Autodesk Inventor part; units mm, degrees
ref_plane "YZ Plane" through (0, 0, 0) normal (1, 0, 0) x (0, 1, 0)
ref_plane "XZ Plane" through (0, 0, 0) normal (0, 1, 0) x (-1, 0, 0)
ref_plane "XY Plane" through (0, 0, 0) normal (0, 0, 1) x (1, 0, 0)
sketch "Sketch1" plane through (0, 0, 0) normal (0, 0, 1) x (1, 0, 0)
  line L0 (0, 0) -> (16, 0)
  line L1 (16, 0) -> (16, 16)
  line L2 (16, 16) -> (0, 16)
  line L3 (0, 16) -> (0, 0)
  dimension "d0" = 16
  dimension "d1" = 16
extrude "Extrusion1" add sketch "Sketch1" along normal blind 12
sketch "Sketch3" plane through (0, 0, 0) normal (0, -1, 0) x (1, 0, 0)
  line L0 (0, 0) -> (16, 0)
  line L1 (0, 0) -> (0, 12)
  circle A0 centre (6, 3) radius 0.75
  circle A1 centre (12.25, 6) radius 3.05
  dimension "d10" = 6.1
  dimension "d11" = 1.5
  dimension "d12" = 3
  dimension "d13" = 6
  dimension "d14" = 6
  dimension "d15" = 12.25
sketch "Sketch2" plane through (0, 0, 12) normal (0, 0, 1) x (1, 0, 0)
  line L0 (0, 16) -> (0, 0)
  circle A0 centre (6, 8) radius 3
  circle A1 centre (13.5, 8) radius 1.4
  point P0 (0, 8)
  dimension "d4" = 13.5
  dimension "d5" = 6
  dimension "d6" = 6
  dimension "d7" = 2.8
chamfer "Chamfer1" distance 0.5 angle 45 12 edges at (0, 0, 6) (8, 0, 12) (0, 8, 12) (8, 16, 12) (0, 16, 6) (0, 8, 0) (8, 16, 0) (8, 0, 0) (16, 8, 0) (16, 8, 12) (16, 0, 6) (16, 16, 6)
extrude "Extrusion4" cut sketch "Sketch3" against normal up to next
extrude "Extrusion5" cut sketch "Sketch2" against normal up to next
thread "Thread1"
thread "Thread2"
properties part number "E3D_Heaterblock"
CAD build for the part. Positions are in the model's coordinates, mm. A direction names the side the tool comes from. Round coordinates to 2 decimals unless told otherwise and drop trailing zeros. Loops run counter-clockwise (first coordinate to the right, second up) from the corner with the lowest first, then second, coordinate; pieces in that order, holes last. Notation, with made-up numbers: M -31.5,15.25 L 25.5,15.25 A23 cw 25.5,49.25 Z; hole C 70.25,15 d1. An arc over 180 degrees is marked long. Use a Markdown table: item, result. Add a question column.
(1) Cut at C-C (y = 11.75). Give the cut face in (x, z), and give its area (3 significant figures).
(2) Cut at D-D (x = 13.5). Give the cut face in (y, z).
(3) Cut at A-A (z = 6). Give the cut face in (x, y), and give its area (3 significant figures).
(4) Which spindle directions (+Z, -Z, +X, -X, +Y, -Y) get a long thin tool onto all of the face, cutting with end or side? Do faces 1 (the face through (16, 8, 6)), 2 (the face through (14.835, 8.421, 10.285)). Say none if no direction does.
(5) Drill centre lines: line 1 (Y direction, x = 6, z = 6.25); line 2 (Z direction, x = 6, y = 3.6); line 3 (Y direction, x = 6.75, z = 2). Where is each one in solid material? Low to high.
(6) Pull direction Y, two halves, no side cores. Call faces 3 (the face through (6, 0, 6)), 4 (the face through (6, 16, 6)), 5 (the face through (7.384, 5.338, 6.084)), 6 (the face through (10, 8, 0)): +Y half, -Y half, draft (parallel to the pull), parting line (faces both ways), or undercut.
(7) Cut at B-B (x = 6). Give the cut face in (y, z).
Geometry says:
| question | item | result |
|---|---|---|
| 1 | outline | M 0,0.5 L 0.5,0 L 15.5,0 L 16,0.5 L 16,11.5 L 15.5,12 L 0.5,12 L 0,11.5 Z; hole C 6,3 d1.5; hole C 12.25,6 d6.1 |
| 1 | area | 161 mm² |
| 2 | outline | M 0,0.5 L 0.5,0 L 15.5,0 L 16,0.5 L 16,3.22 L 0,3.22 Z; M 0,8.78 L 6.6,8.78 L 6.6,12 L 0.5,12 L 0,11.5 Z; M 9.4,8.78 L 16,8.78 L 16,11.5 L 15.5,12 L 9.4,12 Z |
| 3 | outline | M 0,0.5 L 0.5,0 L 9.2,0 L 9.2,16 L 0.5,16 L 0,15.5 Z; M 15.3,0 L 15.5,0 L 16,0.5 L 16,15.5 L 15.5,16 L 15.3,16 Z; hole C 6,8 d6 |
| 3 | area | 130 mm² |
| 4 | face 1 | +Z, -Z, +X, +Y, -Y |
| 4 | face 2 | +Z |
| 5 | line 1 | y = 0 to 5, 11 to 16 |
| 5 | line 2 | z = 0 to 2.25, 3.75 to 12 |
| 5 | line 3 | y = 0 to 5.1, 10.9 to 16 |
| 6 | face 3 | -Y half |
| 6 | face 4 | +Y half |
| 6 | face 5 | undercut |
| 6 | face 6 | draft |
| 7 | outline | M 0,0.5 L 0.5,0 L 5,0 L 5,2.25 L 0,2.25 Z; M 0,3.75 L 5,3.75 L 5,12 L 0.5,12 L 0,11.5 Z; M 11,0 L 15.5,0 L 16,0.5 L 16,2.25 L 11,2.25 Z; M 11,3.75 L 16,3.75 L 16,11.5 L 15.5,12 L 11,12 Z |
